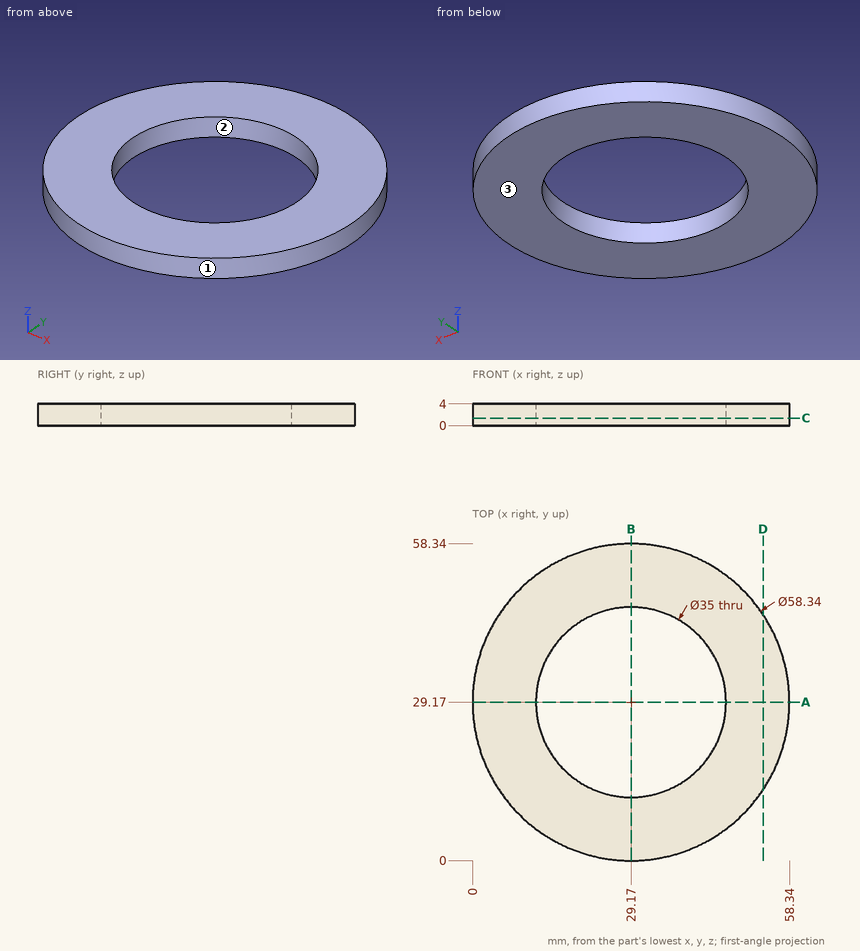
Can you work these out from the drawing? Everything is in mm from the part's minimum corner. Coordinates: 2 decimals unless noted, no trailing zeros. Loops run counter-clockwise (first coordinate to the right, second up) from the corner with the lowest first, then second, coordinate; pieces in that order, holes last. Notation, with made-up numbers: (0, -3.75) - (44, -3.75) arc R25 ccw to (44, 25.25) - close; hole circle Ø10 at (15, 19). An arc over 180 degrees is marked (long way). Put each result on its own line as item: value. Start each with the question number.
Item 1: Suppose I cut it at A-A (y = 29.17). Please give me the cut outline in (x, z).
Item 2: Suppose I cut it at C-C (z = 1.4). Please give me the cut outline in (x, y), and give its area (3 significant figures).
Item 3: For pin 1 (1 mm diameter, centred on x = 27.5, z = 3.5, fed in from +Y); pin 2 (1.5 mm diameter, centred on y = 9.5, z = 3, fed in from -X); pin 3 (1 mm diameter, centred on x = 17.5, z = 2, fed in from -Y), each with a flat end and sliding along its axis, tell me the tip position at first contact or that it passes through.
Item 4: Suppose I cut it at D-D (x = 53.5). Please give me the cut outline in (y, z).
Item 5: If we mould it in two halves opening along X, with no side actions, what happens to the marked faces 1, 2 and 3? For each: +X half, -X half, draft (parallel to the pull), parting line (faces both ways), or undercut.
Item 6: If I drill on line 1 along Y through (x, z) = (29.17, 2.75); line 2 along Y through (x, z) = (36, 0.85); line 3 along X through (y, z) = (45, 3.35), over which ranges is the centre line in solid material (lowest first)?
Here are the results:
1. outline: (0, 0) - (11.67, 0) - (11.67, 4) - (0, 4) - close; (46.67, 0) - (58.34, 0) - (58.34, 4) - (46.67, 4) - close
2. outline: circle Ø58.34 at (29.17, 29.17); hole circle Ø35 at (29.17, 29.17)
2. area: 1,710 mm²
3. pin 1: y = 58.32
3. pin 2: x = 6.97
3. pin 3: y = 2.22
4. outline: (13.08, 0) - (45.26, 0) - (45.26, 4) - (13.08, 4) - close
5. face 1: parting line
5. face 2: undercut
5. face 3: draft
6. line 1: 0 to 11.67, 46.67 to 58.34
6. line 2: 0.81 to 13.06, 45.28 to 57.53
6. line 3: 4.67 to 21.71, 36.63 to 53.67
